Read the model definition and answer for the solid it produces. Units are mm, in the model's axes. A direction names the side the tool comes from. Round coordinates to 2 decimals unless told otherwise and drop trailing zeros. Use one line per item in the form item = value. Start each with the question number.
```python
from build123d import *

# Parameters (mm, degrees)
F0_W     = 18
F0_H     = 4.572
F1_DEPTH = 18
F2_R     = 2.9845
F3_DEPTH = 25.4
F4_R     = 1.75
F5_DEPTH = 25.4
F6_R     = 2.28599


# Not quite as in the source:
# - a fillet or chamfer is up to 0.001 mm smaller than in the source, because OpenCascade refuses the exact size


with BuildPart() as f1:
    # F0 (on Front) → F1 (new body)
    with BuildSketch(Plane.XZ):
        Polygon((5.9780351967, 9.1414450236), (5.9780351967, -3.5585549764), (5.9780351967, -8.1305549764), (10.5500351967, -8.1305549764), (10.5500351967, 9.1414450236), align=None)
        with Locations((-3.0219648033, -5.8445549764)):
            Rectangle(F0_W, F0_H)
    extrude(amount=F1_DEPTH)

    # F2 (on face) → F3 (cut)
    with BuildSketch(Plane.XY.offset(-3.5585549764)):
        with Locations((-3.0219648033, -9)):
            Circle(F2_R)
    extrude(amount=-F3_DEPTH, mode=Mode.SUBTRACT)

    # F4 (on face) → F5 (cut)
    with BuildSketch(Plane.YZ.offset(10.5500351967)):
        with Locations((-14, 5.1414450236)):
            Circle(F4_R)
        with Locations((-4, 5.1414450236)):
            Circle(F4_R)
    extrude(amount=-F5_DEPTH, mode=Mode.SUBTRACT)

    # F6 (radius 2.286 in the source; OpenCascade refuses exactly that, so slightly less here)
    f6_edges = [f1.edges().sort_by_distance(p)[0] for p in [
        (8.264035, -18, 9.141445),
        (8.264035, 0, 9.141445),
        (-12.021965, -18, -5.844555),
        (-12.021965, 0, -5.844555),
        (5.978035, -18, 2.791445),
        (-3.021965, -18, -3.558555),
        (-0.735965, -18, -8.130555),
        (10.550035, -18, 0.505445),
        (5.978035, 0, 2.791445),
        (-3.021965, 0, -3.558555),
        (-0.735965, 0, -8.130555),
        (10.550035, 0, 0.505445),
        (-12.021965, -9, -3.558555),
        (-12.021965, -9, -8.130555),
        (10.550035, -9, -8.130555),
        (10.550035, -9, 9.141445),
        (5.978035, -9, 9.141445),
    ]]
    fillet(f6_edges, radius=F6_R)


solid = f1.part
```
1) Straight lines are drawn through the part: line 1 (Y direction, x = 6.5, z = 3.75); line 2 (Z direction, x = -6.25, y = -5.75); line 3 (X direction, y = -6, z = 3). For each, find the intervals that lie inside material, in ascending order. Write a range as from..to.
2) For faces 4 (the cylindrical face through (6.63, -17.31, 6.17)), 5 (the flat face through (10.55, -9, 0)), 6 (the cylindrical face through (6.63, -0.69, 0.58)), 7 (the flat face through (5.978, -15.4, 6.5)), determine the directions among +Z, -Z, +X, -X, +Y, -Y from which every point of the face is accessible in a straight line to the end or side of a thin tool.
3) Flat-ended cylindrical pins translate along their axes: pin 1 (10.5 mm diameter, centred on x = 0.5, y = -7.5, fed in from +Z); pin 2 (6 mm diameter, centred on x = 3.5, y = -5.5, fed in from +Z); pin 3 (4.5 mm diameter, centred on y = -4, z = 5.14, fed in from -X). Find the tip coordinate at first contact, or state that the pin passes through.
4) Determine the mould class of faces 1 (the cylindrical face through (-3.41, -6.04, -5.81)), 2 (the cylindrical face through (-0.61, -17.35, -7.44)), 3 (the cylindrical face through (6.63, -9.065, 8.454)) for opening direction Y: +Y half, -Y half, draft (parallel to the pull), parting line (faces both ways), or undercut.
Checks:
q1.line_1 = -17.17..-15.06, -12.94..-5.06, -2.94..-0.83
q1.line_2 = -8.13..-3.56
q1.line_3 = 5.98..10.55
q2.face_4 = +Z, -X, -Y
q2.face_5 = +Z, -Z, +X, +Y, -Y
q2.face_6 = +Z, -X, +Y
q2.face_7 = +Z, -X, +Y, -Y
q3.pin_1 = -3.56
q3.pin_2 = 8.31
q3.pin_3 = 5.98
q4.face_1 = undercut
q4.face_2 = -Y half
q4.face_3 = draft
